Input: part model. Units: mm. Frame: model coordinates. Coordinates: 2 decimals unless noted, no trailing zeros. Order: outer loops, then holes, each group sorted by start corner. A loop starts at its lowest first (then second) coordinate and runs counter-clockwise, first axis right, second up. Notation, with made-up numbers: (-8, 53) - (7, 53) arc R18 ccw to (7, 60) - close; hole circle Ø10 at (-21, 10). An arc over 180 degrees is marked (long way). Answer as CSV lines item,"result". Start each with the question number.
Item 1: Section D-D (y = 0.3). Output: boundary loops of the cut face in (x, z).
Item 2: Material intervals for line 1 along X through (y, z) = (0.7, -17); line 2 along Z through (x, y) = (0, 1.15); line 3 along Z through (x, y) = (15, 1.2), sorted ascending.
Item 3: Section B-B (x = 0). Output: boundary loops of the cut face in (y, z).
Item 4: Section A-A (z = 0). Output: boundary loops of the cut face in (x, y), and give its area (3 significant figures).
Item 5: First-contact query: pin 1 (3.5 mm diameter, centred on x = -15, z = -8, fed in from +Y); pin 2 (1.9 mm diameter, centred on x = 15, z = 22, fed in from +Y). Flat tips, straight axial feed; report the tip coordinate or a pass-through.
Item 6: Section C-C (z = -8). Output: boundary loops of the cut face in (x, y), and give its area (3 significant figures).
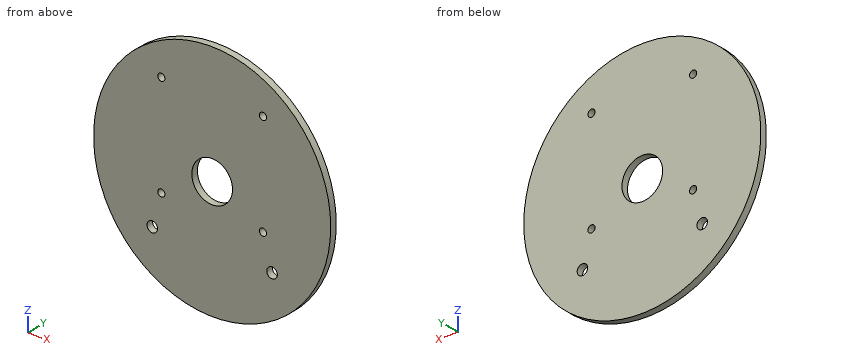
Solid Edge part; units mm, degrees
sketch "Sketch1" plane through (0, 0, 0) normal (0, -1, 0) x (1, 0, 0)
  circle A0 centre (0, 0) radius 35
  circle A1 centre (0, 0) radius 6
extrude "Protrusion1" add sketch "Sketch1" against normal blind 2
sketch "Sketch2" plane through (0, 0, 0) normal (0, -1, 0) x (1, 0, 0)
  circle A0 centre (-15, 22) radius 1.05
  circle A1 centre (-15, -8) radius 1.05
  circle A2 centre (15, 22) radius 1.05
  circle A3 centre (15, -8) radius 1.05
extrude "ExtrudedCutout_4" cut sketch "Sketch2" along normal mid plane 224.2374
sketch "Sketch3" plane through (0, 0, 0) normal (0, -1, 0) x (1, 0, 0)
  circle A0 centre (-17.68, -17.6753) radius 1.55
  circle A1 centre (17.68, -17.6753) radius 1.55
extrude "ExtrudedCutout_5" cut sketch "Sketch3" along normal mid plane 156.4567
Determined:
1,outline,"circle Ø70 at (0, 0); hole circle Ø3.1 at (-17.68, -17.68); hole circle Ø2.1 at (-15, -8); hole circle Ø2.1 at (-15, 22); hole circle Ø12 at (0, 0); hole circle Ø2.1 at (15, -8); hole circle Ø2.1 at (15, 22); hole circle Ø3.1 at (17.68, -17.68)"
2,line 1,"x = -30.59 to -19.08, -16.28 to 16.28, 19.08 to 30.59"
2,line 2,"z = -35 to -6, 6 to 35"
2,line 3,"z = -31.62 to -9.05, -6.95 to 20.95, 23.05 to 31.62"
3,outline,"(0, -35) - (2, -35) - (2, -6) - (0, -6) - close; (0, 6) - (2, 6) - (2, 35) - (0, 35) - close"
4,outline,"(-35, 0) - (-6, 0) - (-6, 2) - (-35, 2) - close; (6, 0) - (35, 0) - (35, 2) - (6, 2) - close"
4,area,"116 mm^2"
5,pin 1,"stops at y = 2"
5,pin 2,"passes through"
6,outline,"(-34.07, 0) - (-16.05, 0) - (-16.05, 2) - (-34.07, 2) - close; (-13.95, 0) - (13.95, 0) - (13.95, 2) - (-13.95, 2) - close; (16.05, 0) - (34.07, 0) - (34.07, 2) - (16.05, 2) - close"
6,area,"128 mm^2"
